Print and shaded views of the part. All mm, measured from the part's lowest x, y and z. Round coordinates to 2 decimals unless told otherwise and drop trailing zeros. Write each loop counter-clockwise with the first axis right and the second up, starting at its lowest first coordinate (ties: lowest second). Pieces come first, ordered by that corner, then holes. Notation, with made-up numbers: M -17.75,-35.75 L 26.25,-35.75 A24 cw 26.25,-20.75 Z; hole C -18,6.25 d7. An arc over 180 degrees is marked long. Write item = value, one per line. Start each with the question number.
Q1. Band-saw the part on D-D on y = 4. Write the cut outline in (x, z).
Q2. Band-saw the part on C-C on z = 6.5. Write the cut outline in (x, y).
Q3. Drop flat-ended pins along their axis: P1, Ø1, axis at x = 12.5, z = 16.5, coming from the -Y side; P2, Ø1, axis at x = 2.5, z = 6, coming from the -Y side; P3, Ø4, axis at x = 15, z = 6, coming from the +Y side. Give the stop position or say it passes through.
Q4. Probe L1, parallel to Y at x = 11, z = 10; L2, parallel to X at y = 10.75, z = 7.75; L3, parallel to Y at x = 9.25, z = 12.5. List the from-to ranges inside material, lowest first.
Q5. Pull direction X, two halves, no side cores. Call the marked faces 1, 2 and 3: released by +X, released by -X, zero draft, split by the parting line, or undercut.
Q6. Band-saw the part on A-A on y = 11. Write the cut outline in (x, z).
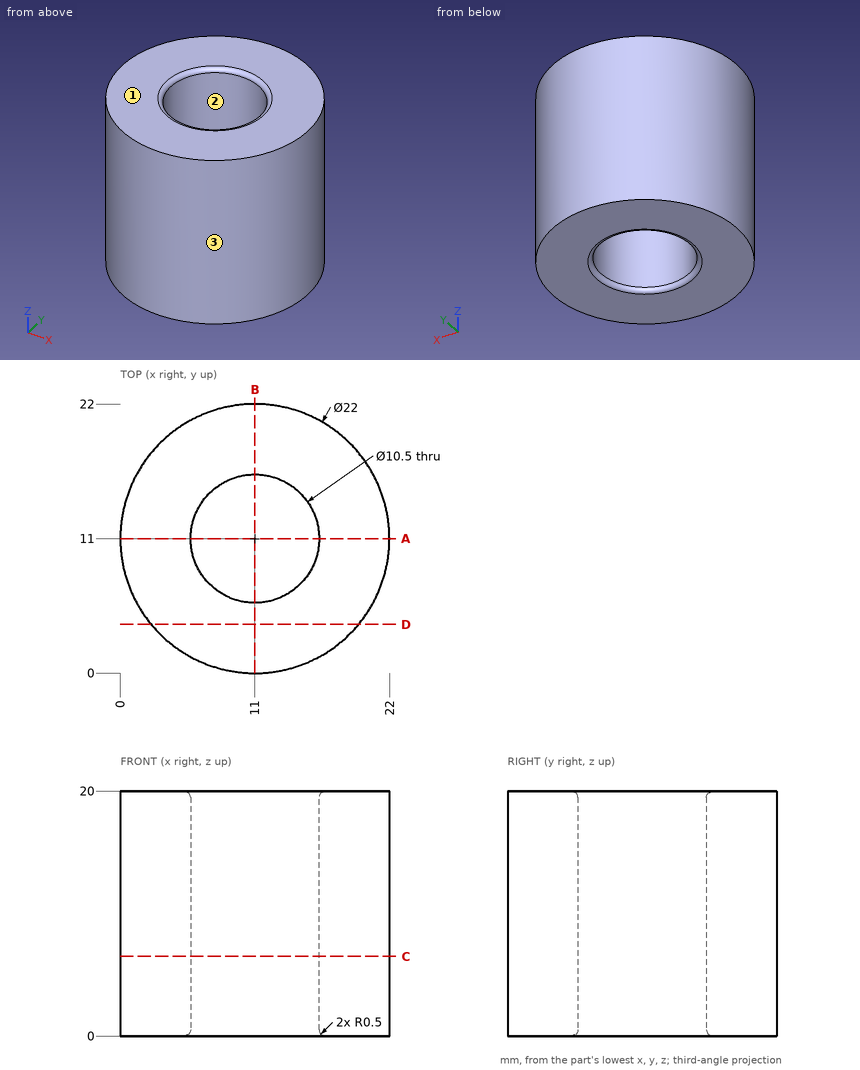
Conclusion:
q1.outline = M 2.51,0 L 19.49,0 L 19.49,20 L 2.51,20 Z
q2.outline = C 11,11 d22; hole C 11,11 d10.5
q3.P1 = 0.05
q3.P2 = 3.45
q3.P3 = 21.82
q4.L1 = 0 to 5.75, 16.25 to 22
q4.L2 = 0 to 5.76, 16.24 to 22
q4.L3 = 0.14 to 6.05, 15.95 to 21.86
q5.face_1 = zero draft
q5.face_2 = undercut
q5.face_3 = split by the parting line
q6.outline = M 0,0 L 5.25,0 A0.5 ccw 5.75,0.5 L 5.75,19.5 A0.5 ccw 5.25,20 L 0,20 Z; M 16.25,0.5 A0.5 ccw 16.75,0 L 22,0 L 22,20 L 16.75,20 A0.5 ccw 16.25,19.5 Z
